Input: part model. Units: mm. Frame: model coordinates. A direction names the side the tool comes from. Give positions to 0.01 mm unless a question says otherwise; leave off trailing zeros. Loops run counter-clockwise (first coordinate to the right, second up) from the corner with the lowest first, then second, coordinate; pieces in that order, holes last. Notation, with made-up numbers: (66.5, -22) -> (72.5, -22) arc R25 ccw to (72.5, -7) -> close; hole circle Ø7 at (3, 41). An arc over 180 degrees is marked (long way). Answer as a JSON object with one key per item and string values. Group by question number.
```python
from build123d import *

# Parameters (mm, degrees)
PAD046_DEPTH    = 4
SKETCH079_R     = 2.85
POCKET030_DEPTH = 5
PAD047_DEPTH    = 10
SKETCH081_R     = 1.15
POCKET031_DEPTH = 5
SKETCH096_W     = 1.6
SKETCH096_H     = 9.4
PAD058_DEPTH    = 8


with BuildPart() as part:
    # Sketch078 → Pad046 (new body)
    with BuildSketch(Plane.YZ):
        with BuildLine():
            Line((0, -13), (45, -13))
            Line((45, -13), (45, 33))
            Line((45, 33), (9, 33))
            ThreePointArc((9, 33), (8.414214, 34.414214), (7, 35))
            Line((7, 35), (3, 35))
            ThreePointArc((3, 35), (0.87868, 34.12132), (0, 32))
            Line((0, 32), (0, -13))
        make_face()
    extrude(amount=PAD046_DEPTH)

    # Sketch079 (on Face9 of Pad046) → Pocket030 (cut)
    with BuildSketch(Plane.YZ.offset(4)):
        with Locations((3.95, 31.05)):
            Circle(SKETCH079_R)
        with BuildLine():
            ThreePointArc((3.5, -6.02), (1.07, -8.45), (3.5, -10.88))
            ThreePointArc((3.5, -10.88), (21.049368, -7.237583), (35.474671, 3.4))
            ThreePointArc((35.474671, 3.4), (35.286946, 6.831408), (31.855538, 6.643683))
            ThreePointArc((3.5, -6.02), (19.067667, -2.800311), (31.855538, 6.643683))
        make_face()
    extrude(amount=-POCKET030_DEPTH, mode=Mode.SUBTRACT)

    # Sketch080 (on Face1 of Pocket030) → Pad047 (join)
    with BuildSketch(Plane.YX.offset(13)):
        Polygon((1.2, 2.1), (5.6, 2.1), (5.6, 10), (7.6, 10), (7.6, 0), (5.6, 0), (1.2, 0), align=None)
    extrude(amount=PAD047_DEPTH)

    # Sketch081 (on Face21 of Pad047) → Pocket031 (cut)
    with BuildSketch(Plane.ZX.offset(7.6)):
        with Locations((-18, 5)):
            Circle(SKETCH081_R)
    extrude(amount=-POCKET031_DEPTH, mode=Mode.SUBTRACT)

    # Sketch096 (on Face6 of Pocket031) → Pad058 (join)
    with BuildSketch(Plane.YZ.offset(4)):
        with Locations((44.2, 25.8)):
            Rectangle(SKETCH096_W, SKETCH096_H)
    extrude(amount=PAD058_DEPTH)


with BuildPart() as part_1:
    # Body019 placement: moved
    add(part.part.moved(Location((-69, -51, -39))))


solid = part_1.part
```
Q1. Pull-direction query (Z, two-part tool) for faces 1 (the face through (-67.03, -42.57, -4.6)), 2 (the face through (-63, -43.4, -56)), 3 (the face through (-66.972, -32.137, -41.891)), 4 (the face through (-61, -7, -17.9)); classes: +Z half, -Z half, draft (parallel to the pull), parting line (faces both ways), or undercut.
Q2. Section D-D on z = -49. Return the cut outline in (x, y), then the cut area to 3 significant figures.
Q3. Section C-C on y = -40. Return the cut outline in (x, z).
Q4. Section B-B on x = -64. Return the cut outline in (y, z).
Q5. Pin query (flat end, axial travel): pin 1 Ø0.8 at (x, y) = (-60.5, -7) entering from +Z; pin 2 Ø5 at (x, z) = (-62.5, -56) entering from +Y; pin 3 Ø6.5 at (x, z) = (-61.5, -56.5) entering from -Y. Return the tip coordinate at first contact, or that it passes through.
Q6. Ray query, probe 1 along Z at (x, y) = (-66.35, -47.05); probe 2 along Z at (x, y) = (-67.75, -47.05); probe 3 along Y at (x, z) = (-66.25, -8). Return the intervals inside material, ascending.
Q7. Set-up query: faces 5 (the face through (-62, -44, -52)), 6 (the face through (-66.97, -30.18, -46.34)), 7 (the face through (-61, -7.6, -13)), 8 (the face through (-67, -25, -52)), 9 (the face through (-62, -45.4, -57)). Return all of +Z, -Z, +X, -X, +Y, -Y with unobstructed straight access to the full face (end or side cutting, diameter ignored); none if empty.
Q8. Section A-A on z = -57. Return the cut outline in (x, y).
Numbers:
{
 "1": {"face 1": "+Z half", "face 2": "draft", "face 3": "undercut", "face 4": "-Z half"},
 "2": {"outline": "(-69, -51) -> (-65, -51) -> (-65, -49.37) -> (-69, -49.37) -> close; (-69, -38.49) -> (-65, -38.49) -> (-65, -6) -> (-69, -6) -> close", "area": "136 mm²"},
 "3": {"outline": "(-69, -52) -> (-65, -52) -> (-65, -49.29) -> (-69, -49.29) -> close; (-69, -44.35) -> (-65, -44.35) -> (-65, -6) -> (-69, -6) -> close"},
 "4": {"outline": "(-45.4, -62) -> (-43.4, -62) -> (-43.4, -58.15) -> (-45.4, -58.15) -> close; (-45.4, -55.85) -> (-43.4, -55.85) -> (-43.4, -52) -> (-45.4, -52) -> close; (-7.6, -17.9) -> (-6, -17.9) -> (-6, -8.5) -> (-7.6, -8.5) -> close"},
 "5": {"pin 1": "stops at z = -8.5", "pin 2": "stops at y = -43.4", "pin 3": "stops at y = -45.4"},
 "6": {"probe 1": "z = -52 to -49.88, -45.02 to -10.8, -5.1 to -4", "probe 2": "z = -62 to -49.88, -45.02 to -10.8, -5.1 to -4", "probe 3": "y = -51 to -49.9, -44.2 to -6"},
 "7": {"face 5": "+Z, +X, +Y, -Y", "face 6": "+X, -X", "face 7": "+Z, -Z, +X, -Y", "face 8": "-Z, +X, -X, +Y", "face 9": "-Z, +X, -Y"},
 "8": {"outline": "(-69, -49.8) -> (-66.9, -49.8) -> (-66.9, -45.4) -> (-65.15, -45.4) -> (-65.15, -43.4) -> (-69, -43.4) -> close; (-62.85, -45.4) -> (-59, -45.4) -> (-59, -43.4) -> (-62.85, -43.4) -> close"}
}
